Work out the finished part from the listing and answer in its coordinate system (mm). Face numbers are marked on the shaded views. A direction names the side the tool comes from. Round coordinates to 2 decimals unless told otherwise and drop trailing zeros. Loops run counter-clockwise (first coordinate to the right, second up) from the corner with the lowest first, then second, coordinate; pieces in that order, holes last. Notation, with made-up numbers: (2, 66) - (15, 66) arc R8 cw to (15, 74) - close; hole circle Ø3 at (35.25, 31). An arc over 180 degrees is marked (long way). Return JSON: item names as keys, results as strings.
from build123d import *

# Parameters (mm, degrees)
SKETCH1_R           = 31.5
BOSS_EXTRUDE1_DEPTH = 5
SKETCH2_R           = 3
CUT_EXTRUDE1_DEPTH  = 11
SKETCH2_4_R         = 2.5
BOSS_EXTRUDE2_DEPTH = 15
SKETCH2_5_R         = 5
CUT_EXTRUDE2_DEPTH  = 6


with BuildPart() as part:
    # Sketch1 → Boss-Extrude1 (new body, symmetric)
    with BuildSketch(Plane.XY):
        Circle(SKETCH1_R)
    extrude(amount=BOSS_EXTRUDE1_DEPTH, both=True)

    # Sketch2 → Cut-Extrude1 (cut, through all)
    with BuildSketch(Plane.XY.offset(5)):
        with Locations((-15, 19.242640687)):
            Circle(SKETCH2_R)
        with Locations((-15, -19.242640687)):
            Circle(SKETCH2_R)
        with Locations((15, -19.242640687)):
            Circle(SKETCH2_R)
        with Locations((15, 19.242640687)):
            Circle(SKETCH2_R)
    extrude(amount=-CUT_EXTRUDE1_DEPTH, mode=Mode.SUBTRACT)

    # Sketch2<4> → Boss-Extrude2 (add)
    with BuildSketch(Plane.XY.offset(5)):
        with Locations((0, 27.5)):
            Circle(SKETCH2_4_R)
    extrude(amount=-BOSS_EXTRUDE2_DEPTH)

    # Sketch2<5> → Cut-Extrude2 (cut)
    with BuildSketch(Plane.XY.offset(5)):
        with Locations((-15, 19.242640687)):
            Circle(SKETCH2_5_R)
        with Locations((-15, -19.242640687)):
            Circle(SKETCH2_5_R)
        with Locations((15, -19.242640687)):
            Circle(SKETCH2_5_R)
        with Locations((15, 19.242640687)):
            Circle(SKETCH2_5_R)
    extrude(amount=-CUT_EXTRUDE2_DEPTH, mode=Mode.SUBTRACT)


solid = part.part
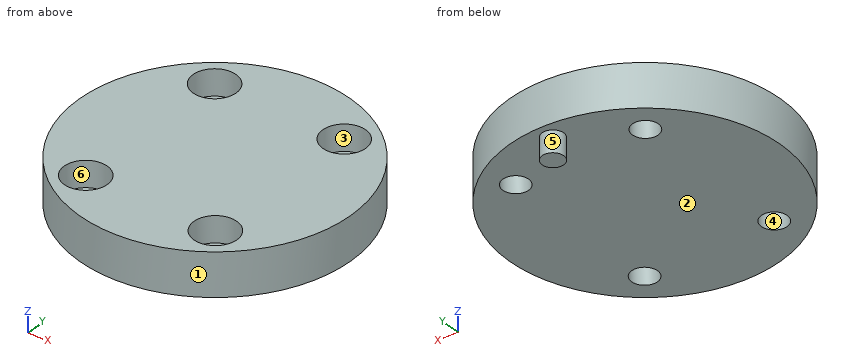
1) Flat-ended cylindrical pins translate along their axes: pin 1 (10 mm diameter, centred on x = 20.5, y = 4.5, fed in from -Z); pin 2 (9 mm diameter, centred on x = -15, y = 19.24, fed in from +Z); pin 3 (5 mm diameter, centred on x = 16.5, y = -17, fed in from +Z); pin 4 (1.5 mm diameter, centred on y = -20.5, z = -5.5, fed in from -X). Find the tip coordinate at first contact, or state that the pin passes through.
Verdict:
{"pin 1": "stops at z = -5", "pin 2": "stops at z = -1", "pin 3": "stops at z = 5", "pin 4": "stops at x = -24.38"}
2) Find the intervals of material crossed by L1, parallel to Y at x = -15, z = 2.55; L2, parallel to Y at x = -15, z = -3.3; L3, parallel to Z at x = 25, y = -2.5, in increasing order.
Verdict:
{"L1": "y = -27.7 to -24.24, -14.24 to 14.24, 24.24 to 27.7", "L2": "y = -27.7 to -22.24, -16.24 to 16.24, 22.24 to 27.7", "L3": "z = -5 to 5"}
3) Section B-B (x = 0) is taken. Give the vertices of the cut face in (y, z), and give its area (3 significant figures).
Verdict:
{"outline": "(-31.5, -5) - (25, -5) - (25, -10) - (30, -10) - (30, -5) - (31.5, -5) - (31.5, 5) - (-31.5, 5) - close", "area": "655 mm2"}
4) Section A-A (x = 15) is taken. Give the vertices of the cut face in (y, z).
Verdict:
{"outline": "(-27.7, -5) - (-22.24, -5) - (-22.24, -1) - (-24.24, -1) - (-24.24, 5) - (-27.7, 5) - close; (-16.24, -5) - (16.24, -5) - (16.24, -1) - (14.24, -1) - (14.24, 5) - (-14.24, 5) - (-14.24, -1) - (-16.24, -1) - close; (22.24, -5) - (27.7, -5) - (27.7, 5) - (24.24, 5) - (24.24, -1) - (22.24, -1) - close"}
5) Section D-D (z = -5.75) is taken. Give the vertices of the cut face in (x, y).
Verdict:
{"outline": "circle Ø5 at (0, 27.5)"}
6) A tool of negligible diameter and unlimited length cuts with its end or side. For the marked faces 4, 5 and 6, from which of +Z, -Z, +X, -X, +Y, -Y can it reach the whole face along a straight path? Write none if from no direction.
Verdict:
{"face 4": "+Z, -Z", "face 5": "-Z", "face 6": "+Z"}
7) Section C-C (y = -18) is taken. Give the vertices of the cut face in (x, z).
Verdict:
{"outline": "(-25.85, -5) - (-17.73, -5) - (-17.73, -1) - (-19.84, -1) - (-19.84, 5) - (-25.85, 5) - close; (-12.27, -5) - (12.27, -5) - (12.27, -1) - (10.16, -1) - (10.16, 5) - (-10.16, 5) - (-10.16, -1) - (-12.27, -1) - close; (17.73, -5) - (25.85, -5) - (25.85, 5) - (19.84, 5) - (19.84, -1) - (17.73, -1) - close"}
8) Determine the mould class of the marked faces 1, 2 and 3 for opening direction Y: pulls with the +Y half, pulls with the -Y half, needs draft (parallel to the pull), parting line crosses it, or undercut.
Verdict:
{"face 1": "parting line crosses it", "face 2": "needs draft", "face 3": "undercut"}
